Source: CAD feature listing. Evaluate the final solid. Frame: model axes, mm. Give positions to 0.01 mm unless a question says otherwise; leave off trailing zeros. Order: outer loops, then holes, each group sorted by start corner. A loop starts at its lowest first (then second) coordinate and runs counter-clockwise, first axis right, second up.
from build123d import *

# Parameters (mm, degrees)
EXTRUDE_1_DEPTH     = 1.5
SKETCH_2_R          = 0.55
CUT_EXTRUDE_1_DEPTH = 1.5
SKETCH_3_R          = 0.4
CUT_EXTRUDE_2_DEPTH = 10
SKETCH_6_R          = 0.465027249
SKETCH_6_R_2        = 0.4
CUT_EXTRUDE_4_DEPTH = 10


with BuildPart() as part:
    # Эскиз1 → Вытянуть1 (new body)
    with BuildSketch(Plane.XY):
        Polygon((0, 20), (0, 25), (40, 25), (40, 20), (50, 20), (50, -20), (-40, -20), (-40, 20), align=None)
    extrude(amount=EXTRUDE_1_DEPTH)

    # Эскиз2 → Вырез-Вытянуть1 (cut)
    with BuildSketch(Plane.XY.offset(1.5)):
        with Locations((-36, 16.54)):
            Circle(SKETCH_2_R)
        with Locations((-36, 11.46)):
            Circle(SKETCH_2_R)
        with Locations((-36, 14)):
            Circle(SKETCH_2_R)
        with Locations((-25.5, -15.5)):
            Circle(SKETCH_2_R)
        with Locations((-25.5, -18.04)):
            Circle(SKETCH_2_R)
        with Locations((-22.96, -15.5)):
            Circle(SKETCH_2_R)
        with Locations((-22.96, -18.04)):
            Circle(SKETCH_2_R)
        with Locations((-20.42, -15.5)):
            Circle(SKETCH_2_R)
        with Locations((-20.42, -18.04)):
            Circle(SKETCH_2_R)
        with Locations((-17.88, -15.5)):
            Circle(SKETCH_2_R)
        with Locations((-17.88, -18.04)):
            Circle(SKETCH_2_R)
        with Locations((-15.34, -15.5)):
            Circle(SKETCH_2_R)
        with Locations((-15.34, -18.04)):
            Circle(SKETCH_2_R)
    extrude(amount=-CUT_EXTRUDE_1_DEPTH, mode=Mode.SUBTRACT)

    # Эскиз3 → Вырез-Вытянуть2 (cut)
    with BuildSketch(Plane.XY.offset(1.5)):
        with Locations((-17.902737838, -8.7)):
            Circle(SKETCH_3_R)
        with Locations((-20.3, 5)):
            Circle(SKETCH_3_R)
        with Locations((8.5, 16.2)):
            Circle(SKETCH_3_R)
        with Locations((8.5, 6.2)):
            Circle(SKETCH_3_R)
        with Locations((11.5, 16.2)):
            Circle(SKETCH_3_R)
        with Locations((11.5, 6.2)):
            Circle(SKETCH_3_R)
        with Locations((14.5, 16.2)):
            Circle(SKETCH_3_R)
        with Locations((14.5, 6.2)):
            Circle(SKETCH_3_R)
        with Locations((17.5, 16.2)):
            Circle(SKETCH_3_R)
        with Locations((17.5, 6.2)):
            Circle(SKETCH_3_R)
        with Locations((20.5, 16.2)):
            Circle(SKETCH_3_R)
        with Locations((20.5, 6.2)):
            Circle(SKETCH_3_R)
        with Locations((23, 16.2)):
            Circle(SKETCH_3_R)
        with Locations((23, 6.2)):
            Circle(SKETCH_3_R)
        with Locations((26, 16.2)):
            Circle(SKETCH_3_R)
        with Locations((26, 6.2)):
            Circle(SKETCH_3_R)
        with Locations((-20.402737838, -8.7)):
            Circle(SKETCH_3_R)
        with Locations((-22.8, 5)):
            Circle(SKETCH_3_R)
        with Locations((-27.8, 6.5)):
            Circle(SKETCH_3_R)
        with Locations((-27.8, 4)):
            Circle(SKETCH_3_R)
    extrude(amount=-CUT_EXTRUDE_2_DEPTH, mode=Mode.SUBTRACT)

    # Эскиз6 → Вырез-Вытянуть4 (cut)
    with BuildSketch(Plane.XY.offset(1.5)):
        with Locations((-28.4, -3.3)):
            Circle(SKETCH_6_R)
        with Locations((-28.4, -0.8)):
            Circle(SKETCH_6_R)
        with Locations((-27.15, -2.05)):
            Circle(SKETCH_6_R)
        with Locations((46.3, 2.5)):
            Circle(SKETCH_6_R_2)
        with Locations((17.5, -13.1)):
            Circle(SKETCH_6_R_2)
        with Locations((44.8, -16)):
            Circle(SKETCH_6_R_2)
    extrude(amount=-CUT_EXTRUDE_4_DEPTH, mode=Mode.SUBTRACT)


solid = part.part
1) Section query A-A on y = 21. Output: boundary loops of the cut face in (x, z).
Checks:
outline: (0, 0) - (40, 0) - (40, 1.5) - (0, 1.5) - close
2) Ray query, L1, parallel to Y at x = -15.34, z = 1.2; L2, parallel to Y at x = 20.5, z = 0.5; L3, parallel to Y at x = -27.15, z = 0.75. Return the intervals inside material, ascending.
Checks:
L1: y = -20 to -18.59, -17.49 to -16.05, -14.95 to 20
L2: y = -20 to 5.8, 6.6 to 15.8, 16.6 to 25
L3: y = -20 to -2.52, -1.58 to 20
3) Section query C-C on x = -33. Output: boundary loops of the cut face in (y, z).
Checks:
outline: (-20, 0) - (20, 0) - (20, 1.5) - (-20, 1.5) - close
4) Section query B-B on z = 0.25. State how many separate pieces and enclosed holes the cut face has, and give its area (3 significant figures).
Checks:
separate pieces: 1
enclosed holes: 39
area: 3,770 mm2
5) First-contact query: pin 1 Ø0.8 at (x, z) = (-14, 0.5) entering from +Y. Flat tip, straight axial feed; report the tip coordinate or a pass-through.
Checks:
pin 1: stops at y = 20
